Autodesk Inventor part; units mm, degrees
ref_plane "YZ Plane" through (0, 0, 0) normal (1, 0, 0) x (0, 1, 0)
ref_plane "XZ Plane" through (0, 0, 0) normal (0, 1, 0) x (-1, 0, 0)
ref_plane "XY Plane" through (0, 0, 0) normal (0, 0, 1) x (1, 0, 0)
sketch "Sketch1" plane through (0, 0, 0) normal (0, 1, 0) x (-1, 0, 0)
  line L0 (9.98, 17.98) -> (-9.98, 17.98)
  line L1 (-9.98, 17.98) -> (-9.98, -17.98)
  line L2 (-9.98, -17.98) -> (9.98, -17.98)
  line L3 (9.98, -17.98) -> (9.98, 17.98)
  line L4 (9.98, 17.98) -> (-9.98, -17.98) construction
  line L5 (-9.98, 17.98) -> (9.98, -17.98) construction
  point P0 (0, 0)
  dimension "d0" = 33.96
  dimension "d1" = 19.96
extrude "arm-wall" add sketch "Sketch1" along normal blind 3
sketch "Sketch2" plane through (0, 3, 0) normal (0, 1, 0) x (1, 0, 0)
  line L0 (-8, -17.98) -> (8, -17.98)
  line L1 (8, -17.98) -> (8, 15.98)
  line L2 (8, 15.98) -> (-8, 15.98)
  line L3 (-8, 15.98) -> (-8, -17.98)
  line L4 (-8, -17.98) -> (8, 15.98) construction
  line L5 (8, -17.98) -> (-8, 15.98) construction
  line L6 (0, 25.172) -> (0, -25.172)
  line L7 (9.98, 17.98) -> (-9.98, 17.98)
  line L8 (-9.98, -17.98) -> (9.98, -17.98)
  point P0 (0, 0)
  point P1 (0, -1)
  point P2 (0, -1)
  dimension "d4" = 16
  dimension "d5" = 1
extrude "slot" cut sketch "Sketch2" against normal blind 2
fillet "Fillet1" radius 2 1 edges at (-9.98, 1.5, 17.98)
fillet "Fillet2" radius 2 1 edges at (9.98, 1.5, 17.98)
fillet "Fillet3" radius 2 1 edges at (9.98, 1.5, -17.98)
fillet "Fillet4" radius 2 1 edges at (-9.98, 1.5, -17.98)
sketch "Sketch3" plane through (0, 0, 0) normal (0, -1, 0) x (1, 0, 0)
  circle A0 centre (0, 0) radius 2.5
  dimension "d12" = 5
extrude "Extrusion3" cut sketch "Sketch3" against normal up to next
equation "\"d2\" = armthick"
equation "\"d4\" = adapterh"
equation "\"d5\" = -0.5 * adapterw + 0.5 * armw"
equation "\"d6\" = armslotd"
equation "\"d8\" = cornerrad"
equation "\"d9\" = cornerrad"
equation "\"d10\" = cornerrad"
equation "\"d11\" = cornerrad"
equation "\"printer3dtolerance\" = 0.1"
equation "\"wallw\" = 42"
equation "\"wallh\" = 44"
equation "\"cornerrad\" = 2"
equation "\"baseextra\" = 2"
equation "\"wall1_thick\" = 8"
equation "\"wall2_thick\" = 6.4"
equation "\"wall3_thick\" = 4"
equation "\"wall1slot\" = 8.1"
equation "\"wall2slot\" = 6.5"
equation "\"wall3slot\" = 4.1"
equation "\"gap2\" = 28"
equation "\"baseh\" = 79"
equation "\"basew\" = 44"
equation "\"base_thick\" = 6"
equation "\"base_slots_depth\" = 4"
equation "\"servobigcircledia\" = 11.6"
equation "\"servosmallcircledia\" = 5.9"
equation "\"servo9gw\" = 22.8"
equation "\"servomounth\" = 4"
equation "\"servomountsquare\" = 4"
equation "\"servopolygonr\" = 6.1"
equation "\"servopolygonl\" = 5.9"
equation "\"distancefrombottom\" = 34"
equation "\"distancefromleft\" = 22"
equation "\"wall3slotd\" = 2"
equation "\"wall3slotw\" = 36"
equation "\"adapterh\" = 16"
equation "\"adapterw\" = 32"
equation "\"armw\" = 34"
equation "\"armslotd\" = 2"
equation "\"armthick\" = 3"
equation "\"fanhb\" = 11"
equation "\"fanhs\" = 9.6"
equation "\"adapterwallslotd\" = 2"
equation "\"adapterwallthick\" = 6"
equation "\"hornscrewholed\" = 2"
equation "\"hornthick\" = 1.5"
equation "\"armhornthick\" = 3"
equation "\"hornscrewheadd\" = 3"
properties part number "slot-wall"
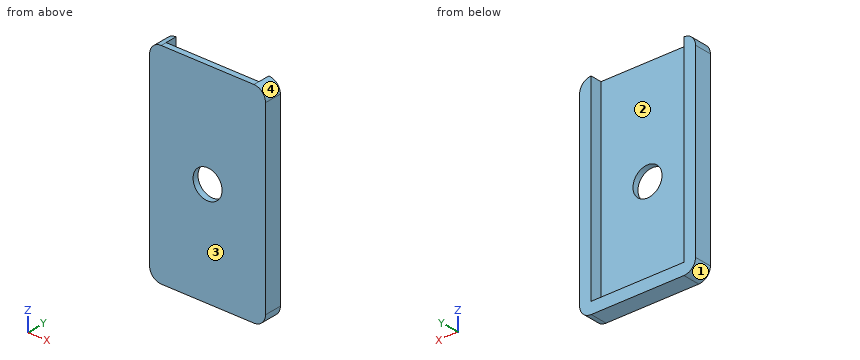
Input: part model. Units: mm. Frame: model coordinates. Face numbers are marked on the shaded views. Coordinates: 2 decimals unless noted, no trailing zeros. Order: outer loops, then holes, each group sorted by start corner. A loop starts at its lowest first (then second) coordinate and runs counter-clockwise, first axis right, second up.
1. Draft query along X for the marked faces 1, 2, 3 and 4. Return one class per face: +X half, -X half, draft (parallel to the pull), parting line (faces both ways), or undercut.
Checked values:
face 1: -X half
face 2: undercut
face 3: draft
face 4: +X half
2. Ray query, line 1 along X through (y, z) = (1.6, -7); line 2 along Z through (x, y) = (0, 0.2); line 3 along Y through (x, z) = (-1.75, 5.5). Return the intervals inside material, ascending.
Checked values:
line 1: x = -9.98 to -8, 8 to 9.98
line 2: z = -17.98 to -2.5, 2.5 to 17.98
line 3: y = 0 to 1
3. Cut plane A-A, the plane z = 0. Return loops of the section in (x, y).
Checked values:
outline: (-9.98, 0) - (-2.5, 0) - (-2.5, 1) - (-8, 1) - (-8, 3) - (-9.98, 3) - close; (2.5, 0) - (9.98, 0) - (9.98, 3) - (8, 3) - (8, 1) - (2.5, 1) - close
4. Cut plane C-C, the plane y = 0.6. Return loops of the section in (x, z), plus the area to 3 significant figures.
Checked values:
outline: (-9.98, -15.98) arc R2 ccw to (-7.98, -17.98) - (7.98, -17.98) arc R2 ccw to (9.98, -15.98) - (9.98, 15.98) arc R2 ccw to (7.98, 17.98) - (-7.98, 17.98) arc R2 ccw to (-9.98, 15.98) - close; hole circle Ø5 at (0, 0)
area: 695 mm2
5. Cut plane B-B, the plane x = 0. Return loops of the section in (y, z).
Checked values:
outline: (0, -17.98) - (3, -17.98) - (3, -15.98) - (1, -15.98) - (1, -2.5) - (0, -2.5) - close; (0, 2.5) - (1, 2.5) - (1, 17.98) - (0, 17.98) - close
6. Contact query for flat-ended pins moving along their axis: P1, Ø8, axis at x = -1.5, z = -4.5, coming from the +Y side; P2, Ø1.6, axis at x = 2, y = 2, coming from the +Z side. Output: stop coordinate, or through.
Checked values:
P1: stops at y = 1
P2: stops at z = -15.98
